Here's how the part is built. I have some questions about the finished solid (model axes, mm). A direction names the side the tool comes from. Coordinates: 2 decimals unless noted, no trailing zeros. Write each loop counter-clockwise with the first axis right and the second up, starting at its lowest first coordinate (ties: lowest second). Pieces come first, ordered by that corner, then holes. Notation, with made-up numbers: (6.25, 23.25) -> (28.25, 23.25) arc R26 ccw to (28.25, 40.25) -> close; hole circle Ø4 at (63.25, 43). An arc over 180 degrees is marked (long way). Answer in a Markdown table with one row per item. Add a question column.
from build123d import *

# Parameters (mm, degrees)
SKETCH_1_W          = 388
SKETCH_1_H          = 100
EXTRUDE_1_DEPTH     = 420
SKETCH_2_W          = 20
SKETCH_2_H          = 420
EXTRUDE_2_DEPTH     = 30
SKETCH_3_W          = 20
SKETCH_3_H          = 20
EXTRUDE_3_DEPTH     = 500
SKETCH_4_W          = 388
SKETCH_4_H          = 420
EXTRUDE_4_DEPTH     = 20
SKETCH_6_W          = 308
SKETCH_6_H          = 290
EXTRUDE_6_DEPTH     = 10
CUT_EXTRUDE_1_REACH = 802.555
CUT_EXTRUDE_2_REACH = 845.412
SKETCH_8_W          = 348
SKETCH_8_H          = 380
SKETCH_9_W          = 45
SKETCH_9_H          = 20
EXTRUDE_7_DEPTH     = 25
SKETCH_10_W         = 45
SKETCH_10_H         = 20
EXTRUDE_8_DEPTH     = 25


with BuildPart() as part:
    # 草图1 → 凸台-拉伸1 (new body)
    with BuildSketch(Plane.XY):
        with Locations((194, 50)):
            Rectangle(SKETCH_1_W, SKETCH_1_H)
    extrude(amount=-EXTRUDE_1_DEPTH)

    # 草图2 → 凸台-拉伸2 (add)
    with BuildSketch(Plane(origin=(0, 100, 0), x_dir=(1, 0, 0), z_dir=(0, 1, 0))):
        with Locations((115, 210)):
            Rectangle(SKETCH_2_W, SKETCH_2_H)
        with Locations((273, 210)):
            Rectangle(SKETCH_2_W, SKETCH_2_H)
    extrude(amount=EXTRUDE_2_DEPTH)

    # 草图3 → 凸台-拉伸3 (add)
    with BuildSketch(Plane(origin=(0, 100, 0), x_dir=(1, 0, 0), z_dir=(0, 1, 0))):
        with Locations((10, 10)):
            Rectangle(SKETCH_3_W, SKETCH_3_H)
        with Locations((10, 410)):
            Rectangle(SKETCH_3_W, SKETCH_3_H)
        with Locations((378, 10)):
            Rectangle(SKETCH_3_W, SKETCH_3_H)
        with Locations((378, 410)):
            Rectangle(SKETCH_3_W, SKETCH_3_H)
    extrude(amount=EXTRUDE_3_DEPTH)

    # 草图4 → 凸台-拉伸4 (add)
    with BuildSketch(Plane(origin=(0, 600, 0), x_dir=(1, 0, 0), z_dir=(0, 1, 0))):
        with Locations((194, 210)):
            Rectangle(SKETCH_4_W, SKETCH_4_H)
    extrude(amount=EXTRUDE_4_DEPTH)

    # 草图6 → 凸台-拉伸6 (add)
    with BuildSketch(Plane(origin=(0, 130, 0), x_dir=(1, 0, 0), z_dir=(0, 1, 0))):
        with Locations((194, 175)):
            Rectangle(SKETCH_6_W, SKETCH_6_H)
    extrude(amount=EXTRUDE_6_DEPTH)

    # 切除-拉伸1: up to this face of the body (flat: up to its plane)
    cut_extrude_1_end = Plane(part.part.faces().sort_by_distance((283, 115, -210))[0])
    # 草图7 → 切除-拉伸1 (cut, up to the picked face)
    with BuildSketch(Plane.ZY.offset(-105), mode=Mode.PRIVATE) as cut_extrude_1_sk1:
        Polygon((0, 100), (-20, 130), (0, 130), align=None)
    cut_extrude_1_tool1 = split(extrude(cut_extrude_1_sk1.sketch, amount=-CUT_EXTRUDE_1_REACH, mode=Mode.PRIVATE), bisect_by=cut_extrude_1_end, keep=Keep.BOTH, mode=Mode.PRIVATE)
    add(cut_extrude_1_tool1.solids().sort_by(Axis((105, 120, -6.666667), (1, 0, 0)))[0], mode=Mode.SUBTRACT)

    # 草图8 → 切除-拉伸2 (cut, up to next)
    with BuildSketch(Plane(origin=(0, 620, 0), x_dir=(1, 0, 0), z_dir=(0, 1, 0)), mode=Mode.PRIVATE) as cut_extrude_2_sk1:
        with Locations((194, 210)):
            Rectangle(SKETCH_8_W, SKETCH_8_H)
    cut_extrude_2_tool1 = extrude(cut_extrude_2_sk1.sketch, amount=-CUT_EXTRUDE_2_REACH, mode=Mode.PRIVATE) & part.part
    add(cut_extrude_2_tool1.solids().sort_by_distance((194, 620, -210))[0], mode=Mode.SUBTRACT)

    # 草图9 → 凸台-拉伸7 (add)
    with BuildSketch(Plane.ZY.offset(-368)):
        with Locations((-42.5, 610)):
            Rectangle(SKETCH_9_W, SKETCH_9_H)
        with Locations((-377.5, 610)):
            Rectangle(SKETCH_9_W, SKETCH_9_H)
    extrude(amount=EXTRUDE_7_DEPTH)

    # 草图10 → 凸台-拉伸8 (add)
    with BuildSketch(Plane(origin=(20, 0, 0), x_dir=(0, 0, -1), z_dir=(1, 0, 0))):
        with Locations((377.5, 610)):
            Rectangle(SKETCH_10_W, SKETCH_10_H)
        with Locations((42.5, 610)):
            Rectangle(SKETCH_10_W, SKETCH_10_H)
    extrude(amount=EXTRUDE_8_DEPTH)


solid = part.part
Q1. Imagine slicing it at C-C on z = -261. Please give me the cut outline in (x, y).
Q2. If we mould it in two halves opening along X, with no side actions, what happens to faces 5 (the flat face through (265, 125, -420)), 6 (the flat face through (388, 79, -209)), 7 (the flat face through (32, 610, -355)), 8 (the flat face through (20, 346, -10))? For each: pulls with the +X half, pulls with the -X half, needs draft (parallel to the pull), parting line crosses it, or undercut.
Q3. Imagine slicing it at D-D on y = 504. Please give me the cut outline in (x, z), plus the area to 3 significant figures.
Q4. I need wall thicknesses on line 1 (Y direction, x = 311.5, z = -191.5); line 2 (X direction, y = 125.5, z = -355.5); line 3 (Z direction, x = 370, y = 491.5). Which ranges of each line are inside material? Lowest first, please. Write a range as [from, to].
Q5. For faces 1 (the flat face through (115, 130, -371)), 2 (the flat face through (380, 620, -193)), 3 (the flat face through (45, 610, -42)), 4 (the flat face through (125, 115, -207)), which set-ups out of +Z, -Z, +X, -X, +Y, -Y let a thin tool reach every point of the face, with its end or its side?
Q6. I'm going to push flat-ended pins straight in: P1, Ø6, axis at x = 278, z = -251.5, coming from the +Y side; P2, Ø24, axis at y = 121.5, z = -288, coming from the +X side; P3, Ø6, axis at x = 276.5, z = -345.5, coming from the +Y side. Where does each tip first touch, or does it pass through?
Q7. Imagine slicing it at B-B on x = 63. Please give me the cut outline in (y, z).
Q8. Imagine slicing it at A-A on z = -389. Please give me the cut outline in (x, y).
Result sheet:
| question | item | result |
|---|---|---|
| 1 | outline | (0, 0) -> (388, 0) -> (388, 100) -> (283, 100) -> (283, 130) -> (348, 130) -> (348, 140) -> (40, 140) -> (40, 130) -> (105, 130) -> (105, 100) -> (0, 100) -> close; (0, 600) -> (20, 600) -> (20, 620) -> (0, 620) -> close; (368, 600) -> (388, 600) -> (388, 620) -> (368, 620) -> close; hole (125, 100) -> (263, 100) -> (263, 130) -> (125, 130) -> close |
| 2 | face 5 | needs draft |
| 2 | face 6 | pulls with the +X half |
| 2 | face 7 | undercut |
| 2 | face 8 | undercut |
| 3 | outline | (0, -420) -> (20, -420) -> (20, -400) -> (0, -400) -> close; (0, -20) -> (20, -20) -> (20, 0) -> (0, 0) -> close; (368, -420) -> (388, -420) -> (388, -400) -> (368, -400) -> close; (368, -20) -> (388, -20) -> (388, 0) -> (368, 0) -> close |
| 3 | area | 1,600 mm^2 |
| 4 | line 1 | y = [0, 100], [130, 140] |
| 4 | line 2 | x = [105, 125], [263, 283] |
| 4 | line 3 | z = [-420, -400], [-20, 0] |
| 5 | face 1 | -Z |
| 5 | face 2 | +Z, -Z, +X, -X, +Y |
| 5 | face 3 | +Y |
| 5 | face 4 | +Z, -Z |
| 6 | P1 | stops at y = 140 |
| 6 | P2 | stops at x = 348 |
| 6 | P3 | stops at y = 130 |
| 7 | outline | (0, -420) -> (100, -420) -> (100, 0) -> (0, 0) -> close; (130, -320) -> (140, -320) -> (140, -30) -> (130, -30) -> close; (600, -420) -> (620, -420) -> (620, -400) -> (600, -400) -> close; (600, -20) -> (620, -20) -> (620, 0) -> (600, 0) -> close |
| 8 | outline | (0, 0) -> (388, 0) -> (388, 100) -> (283, 100) -> (283, 130) -> (263, 130) -> (263, 100) -> (125, 100) -> (125, 130) -> (105, 130) -> (105, 100) -> (0, 100) -> close; (0, 600) -> (45, 600) -> (45, 620) -> (0, 620) -> close; (343, 600) -> (388, 600) -> (388, 620) -> (343, 620) -> close |
